from build123d import *

# Parameters (mm, degrees)
F1_DEPTH = 1
F2_W     = 27.3
F2_H     = 19
F3_DEPTH = 1
F4_W     = 27.3
F4_H     = 15
F5_DEPTH = 0.01


with BuildPart() as f1:
    # F0 (on Top) → F1 (new body)
    with BuildSketch(Plane.XY):
        with BuildLine():
            Line((-11.65, -13.65), (11.65, -13.65))
            ThreePointArc((11.65, -13.65), (13.064214, -13.064214), (13.65, -11.65))
            Line((13.65, -11.65), (13.65, 11.65))
            ThreePointArc((13.65, 11.65), (13.064214, 13.064214), (11.65, 13.65))
            Line((11.65, 13.65), (-11.65, 13.65))
            ThreePointArc((-11.65, 13.65), (-13.064214, 13.064214), (-13.65, 11.65))
            Line((-13.65, 11.65), (-13.65, -11.65))
            ThreePointArc((-13.65, -11.65), (-13.064214, -13.064214), (-11.65, -13.65))
        make_face()
        with BuildLine():
            Line((-9.85, -12.85), (-10.85, -12.85))
            ThreePointArc((-10.85, -12.85), (-11.733883, -12.483883), (-12.1, -11.6))
            ThreePointArc((-12.1, -11.6), (-11.733883, -10.716117), (-10.85, -10.35))
            Line((-10.85, -10.35), (-9.85, -10.35))
            ThreePointArc((-9.85, -10.35), (-8.966117, -10.716117), (-8.6, -11.6))
            ThreePointArc((-8.6, -11.6), (-8.966117, -12.483883), (-9.85, -12.85))
        make_face(mode=Mode.SUBTRACT)
        with BuildLine():
            ThreePointArc((8.6, -11.6), (8.966117, -10.716117), (9.85, -10.35))
            Line((9.85, -10.35), (10.85, -10.35))
            ThreePointArc((10.85, -10.35), (11.733883, -10.716117), (12.1, -11.6))
            ThreePointArc((12.1, -11.6), (11.733883, -12.483883), (10.85, -12.85))
            Line((10.85, -12.85), (9.85, -12.85))
            ThreePointArc((9.85, -12.85), (8.966117, -12.483883), (8.6, -11.6))
        make_face(mode=Mode.SUBTRACT)
        with BuildLine():
            ThreePointArc((-8.6, 11.6), (-8.966117, 10.716117), (-9.85, 10.35))
            Line((-9.85, 10.35), (-10.85, 10.35))
            ThreePointArc((-10.85, 10.35), (-11.733883, 10.716117), (-12.1, 11.6))
            ThreePointArc((-12.1, 11.6), (-11.733883, 12.483883), (-10.85, 12.85))
            Line((-10.85, 12.85), (-9.85, 12.85))
            ThreePointArc((-9.85, 12.85), (-8.966117, 12.483883), (-8.6, 11.6))
        make_face(mode=Mode.SUBTRACT)
        with BuildLine():
            ThreePointArc((8.6, 11.6), (8.966117, 12.483883), (9.85, 12.85))
            Line((9.85, 12.85), (10.85, 12.85))
            ThreePointArc((10.85, 12.85), (11.733883, 12.483883), (12.1, 11.6))
            ThreePointArc((12.1, 11.6), (11.733883, 10.716117), (10.85, 10.35))
            Line((10.85, 10.35), (9.85, 10.35))
            ThreePointArc((9.85, 10.35), (8.966117, 10.716117), (8.6, 11.6))
        make_face(mode=Mode.SUBTRACT)
    extrude(amount=F1_DEPTH)

    # F2 (on face) → F3 (join)
    with BuildSketch(Plane.XY.offset(1)):
        Rectangle(F2_W, F2_H)
    extrude(amount=F3_DEPTH)

    # F4 (on face) → F5 (join)
    with BuildSketch(Plane.XY.offset(2)):
        with Locations((0, 2)):
            Rectangle(F4_W, F4_H)
    extrude(amount=F5_DEPTH)


solid = f1.part
The model under review builds one solid part; all positions refer to its coordinate system, in mm. A direction names the side the tool comes from. Give positions to 0.01 mm unless a question says otherwise; leave off trailing zeros. Answer in a Markdown table with one row per item. Add a question column.
1. Machinability: for faces 4 (the flat face through (-0.2, -9.5, 1.5)), 5 (the flat face through (10.3, -10.35, 0.5)), 6 (the cylindrical face through (13.05, -13.08, 0.49)), which of the approach directions +Z, -Z, +X, -X, +Y, -Y give a long, thin tool a straight path to every point of the face, cutting with its end or side? Answer none if there is none.
2. Add section A-A on z = 0.55. Count the separate pieces of the cut face and the enclosed holes in it, plus the area to 3 significant figures.
3. For pin 1 Ø1.2 at (x, y) = (0.5, 11) entering from +Z; pin 2 Ø1.2 at (x, y) = (4.5, -8) entering from +Z; pin 3 Ø0.5 at (x, z) = (2, 1.5) entering from +Y, all flat-tipped, find the tip position at first contact; note any pin that passes through.
4. Mouldability with a two-part tool opening along Y and no side actions: class faces 1 (the flat face through (10.4, 10.35, 0.5)), 2 (the flat face through (-0.2, 9.5, 1.5)), 3 (the flat face through (0, 0, 0)) as released by +Y, released by -Y, zero draft, split by the parting line, or undercut.
5. To check wall thickness, follow line 1 along Y through (x, z) = (9.5, 1.9); line 2 along Z through (x, y) = (-7.5, -9.25); line 3 along Z through (x, y) = (8, -10). State the ranges of each line that lie inside material, in increasing order.
The answers:
| question | item | result |
|---|---|---|
| 1 | face 4 | +Z, +X, -X, -Y |
| 1 | face 5 | +Z, -Z |
| 1 | face 6 | +Z, -Z, +X, -Y |
| 2 | separate pieces | 1 |
| 2 | enclosed holes | 4 |
| 2 | area | 712 mm2 |
| 3 | pin 1 | z = 1 |
| 3 | pin 2 | z = 2 |
| 3 | pin 3 | y = 9.5 |
| 4 | face 1 | undercut |
| 4 | face 2 | released by +Y |
| 4 | face 3 | zero draft |
| 5 | line 1 | -9.5 to 9.5 |
| 5 | line 2 | 0 to 2 |
| 5 | line 3 | 0 to 1 |
